Build history of the part. All positions in model axes, mm. Round coordinates to 2 decimals unless told otherwise and drop trailing zeros. Write each loop counter-clockwise with the first axis right and the second up, starting at its lowest first coordinate (ties: lowest second). Pieces come first, ordered by that corner, then holes. Notation, with made-up numbers: (-37, 55) - (-2, 55) arc R22 cw to (-2, 93) - close; hole circle Ø4 at (-32.75, -27.75). An arc over 180 degrees is marked (long way). Write each question's results on one line, items separated by ' | '.
from build123d import *

# Parameters (mm, degrees)
F0_R     = 2.7
F0_R_2   = 1.7
F0_R_3   = 11
F1_DEPTH = 8


with BuildPart() as f1:
    # F0 (on Front) → F1 (new body)
    with BuildSketch(Plane.XZ):
        with BuildLine():
            ThreePointArc((-18, 17.5), (-19.414214, 16.914214), (-20, 15.5))
            Line((-20, 15.5), (-20, -35.7))
            ThreePointArc((-20, -35.7), (-19.414214, -37.114214), (-18, -37.7))
            Line((-18, -37.7), (18, -37.7))
            ThreePointArc((18, -37.7), (19.414214, -37.114214), (20, -35.7))
            Line((20, -35.7), (20, 15.5))
            ThreePointArc((20, 15.5), (19.414214, 16.914214), (18, 17.5))
            Line((18, 17.5), (-18, 17.5))
        make_face()
        with Locations((-10, -27.7)):
            Circle(F0_R, mode=Mode.SUBTRACT)
        with Locations((-14.5, -14.5)):
            Circle(F0_R_2, mode=Mode.SUBTRACT)
        with Locations((10, -27.7)):
            Circle(F0_R, mode=Mode.SUBTRACT)
        with Locations((14.5, -14.5)):
            Circle(F0_R_2, mode=Mode.SUBTRACT)
        with Locations((-14.5, 14.5)):
            Circle(F0_R_2, mode=Mode.SUBTRACT)
        Circle(F0_R_3, mode=Mode.SUBTRACT)
        with Locations((14.5, 14.5)):
            Circle(F0_R_2, mode=Mode.SUBTRACT)
    extrude(amount=-F1_DEPTH)


solid = f1.part
(1) Two-plate mould, pull along Z, no slides. Class faces 1 (the flat face through (0, 0, -16)), 2 (the cylindrical face through (19.4, 3.94, -37.13)), 3 (the cylindrical face through (-2.38, 3.94, -10.74)): released by +Z, released by -Z, zero draft, split by the parting line, or undercut.
Worked answers:
face 1: zero draft | face 2: released by -Z | face 3: undercut
(2) Slice it at A-A, the plane y = 4.75. Write the cut outline in (x, z).
Worked answers:
outline: (-20, -35.7) arc R2 ccw to (-18, -37.7) - (18, -37.7) arc R2 ccw to (20, -35.7) - (20, 15.5) arc R2 ccw to (18, 17.5) - (-18, 17.5) arc R2 ccw to (-20, 15.5) - close; hole circle Ø3.4 at (-14.5, -14.5); hole circle Ø3.4 at (-14.5, 14.5); hole circle Ø5.4 at (-10, -27.7); hole circle Ø22 at (0, 0); hole circle Ø5.4 at (10, -27.7); hole circle Ø3.4 at (14.5, -14.5); hole circle Ø3.4 at (14.5, 14.5)
(3) Drill centre lines: probe 1 along Z at (x, y) = (14.5, 1.5); probe 2 along Z at (x, y) = (0, 4.5); probe 3 along Z at (x, y) = (10, 3.5). Where is each one in solid material? Low to high. Write a range as [from, to].
Worked answers:
probe 1: z = [-37.7, -16.2], [-12.8, 12.8], [16.2, 17.5] | probe 2: z = [-37.7, -11], [11, 17.5] | probe 3: z = [-37.7, -30.4], [-25, -4.58], [4.58, 17.5]
(4) Slice it at B-B, the plane z = -27.7. Write the cut outline in (x, y).
Worked answers:
outline: (-20, 0) - (-12.7, 0) - (-12.7, 8) - (-20, 8) - close; (-7.3, 0) - (7.3, 0) - (7.3, 8) - (-7.3, 8) - close; (12.7, 0) - (20, 0) - (20, 8) - (12.7, 8) - close
(5) Flat gauge pin, fed straight in: pin 1 Ø2 at (x, z) = (14.5, 14.5) entering from +Y. Where does the tip first touch, or does it go through?
Worked answers:
pin 1: passes through
(6) Slice it at C-C, the plane z = -5.5. Write the cut outline in (x, y), and give its area (3 significant figures).
Worked answers:
outline: (-20, 0) - (-9.53, 0) - (-9.53, 8) - (-20, 8) - close; (9.53, 0) - (20, 0) - (20, 8) - (9.53, 8) - close | area: 168 mm2
(7) Slice it at D-D, the plane x = 4. Write the cut outline in (y, z), and give its area (3 significant figures).
Worked answers:
outline: (0, -37.7) - (8, -37.7) - (8, -10.25) - (0, -10.25) - close; (0, 10.25) - (8, 10.25) - (8, 17.5) - (0, 17.5) - close | area: 278 mm2
